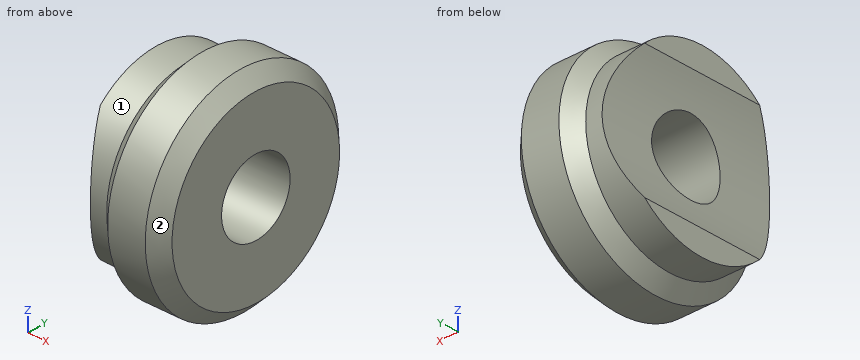
```python
from build123d import *

# Parameters (mm, degrees)
ESBO_O2_R                  = 8.5
CORTE_EXTRUS_O1_DEPTH      = 7.35
CORTE_EXTRUS_O1_DEPTH_BACK = 7.35


with BuildPart() as part:
    # Esboço1 → Revolução1 (revolve)
    with BuildSketch(Plane.XY):
        Polygon((0, 5.5), (2, 5.5), (2.85, 6.35), (5.15, 6.35), (6, 5.5), (6, 2.25), (0.692820323, 2.25), (0, 2.65), align=None)
    revolve(axis=Axis((14.266397253, 0, 0), (1, 0, 0)))

    # Esboço2 → Corte-extrusão1 (cut, two sides)
    with BuildSketch(Plane(origin=(0, 0, 0), x_dir=(1, 0, 0), z_dir=(0, 1, 0))) as corte_extrus_o1_sk:
        with Locations((-7.5, 0)):
            Circle(ESBO_O2_R)
    extrude(amount=CORTE_EXTRUS_O1_DEPTH, mode=Mode.SUBTRACT)
    extrude(corte_extrus_o1_sk.sketch, amount=-CORTE_EXTRUS_O1_DEPTH_BACK, mode=Mode.SUBTRACT)


solid = part.part
```
Read the model definition and answer for the solid it produces. Units are mm, in the model's axes. Face numbers are marked on the shaded views. A direction names the side the tool comes from. Coordinates: 2 decimals unless noted, no trailing zeros. Write each loop counter-clockwise with the first axis right and the second up, starting at its lowest first coordinate (ties: lowest second). Pieces come first, ordered by that corner, then holes. Notation, with made-up numbers: (-15.5, 72.5) -> (-10.5, 72.5) arc R27 ccw to (-10.5, 103.5) -> close; hole circle Ø2 at (-21, 61.25). An arc over 180 degrees is marked (long way). Write item = value, one per line.
(1) Given pin 1 Ø5 at (y, z) = (0, 0) entering from +X; pin 2 Ø1.5 at (x, y) = (2, 0.5) entering from -Z, each flat-ended and moving along its own axis, determine where each tip first touches the part or whether it passes through.
From the geometry:
pin_1 = 6
pin_2 = -6.23
(2) Section D-D on x = 3.25 is taken. Write down the section's boundary in (y, z).
From the geometry:
outline = circle Ø12.7 at (0, 0); hole circle Ø4.5 at (0, 0)
(3) Which of the six approach directions +Z, -Z, +X, -X, +Y, -Y give full straight-line access (tool end or side, diameter ignored) to the marked faces 1 and 2?
From the geometry:
face_1 = -X
face_2 = +X
(4) Straight lines are drawn through the part: L1, parallel to Z at x = 1.95, y = 0; L2, parallel to Z at x = 3.3, y = 0. For each, find the intervals that lie inside material, in ascending order. Write a range as from..to.
From the geometry:
L1 = -5.5..-2.25, 2.25..5.5
L2 = -6.35..-2.25, 2.25..6.35
(5) Section C-C on x = 2.5 is taken. Write down the section's boundary in (y, z), plus the area to 3 significant figures.
From the geometry:
outline = circle Ø12 at (0, 0); hole circle Ø4.5 at (0, 0)
area = 97.2 mm2
(6) Section A-A on y = 0 is taken. Write down the section's boundary in (x, z).
From the geometry:
outline = (0, -5.5) -> (2, -5.5) -> (2.85, -6.35) -> (5.15, -6.35) -> (6, -5.5) -> (6, -2.25) -> (0.7, -2.25) arc R8.5 cw to (0, -4) -> close; (0, 4) arc R8.5 cw to (0.7, 2.25) -> (6, 2.25) -> (6, 5.5) -> (5.15, 6.35) -> (2.85, 6.35) -> (2, 5.5) -> (0, 5.5) -> close
(7) Section B-B on z = 0 is taken. Write down the section's boundary in (x, y).
From the geometry:
outline = (1, -5.5) -> (2, -5.5) -> (2.85, -6.35) -> (5.15, -6.35) -> (6, -5.5) -> (6, -2.25) -> (1, -2.25) -> close; (1, 2.25) -> (6, 2.25) -> (6, 5.5) -> (5.15, 6.35) -> (2.85, 6.35) -> (2, 5.5) -> (1, 5.5) -> close
